Answer from the drawing. Dimensions are ordinates in mm from the lowest x, y and z of the part. Round coordinates to 2 decimals unless told otherwise and drop trailing zeros. Loops run counter-clockwise (first coordinate to the right, second up) from the corner with the lowest first, then second, coordinate; pieces in that order, holes last. Notation, with made-up numbers: (7, 26) - (50, 26) arc R29 cw to (50, 53) - close; hole circle Ø3 at (81, -10.5). An arc over 180 degrees is marked (long way). Answer as CSV lines item,"result".
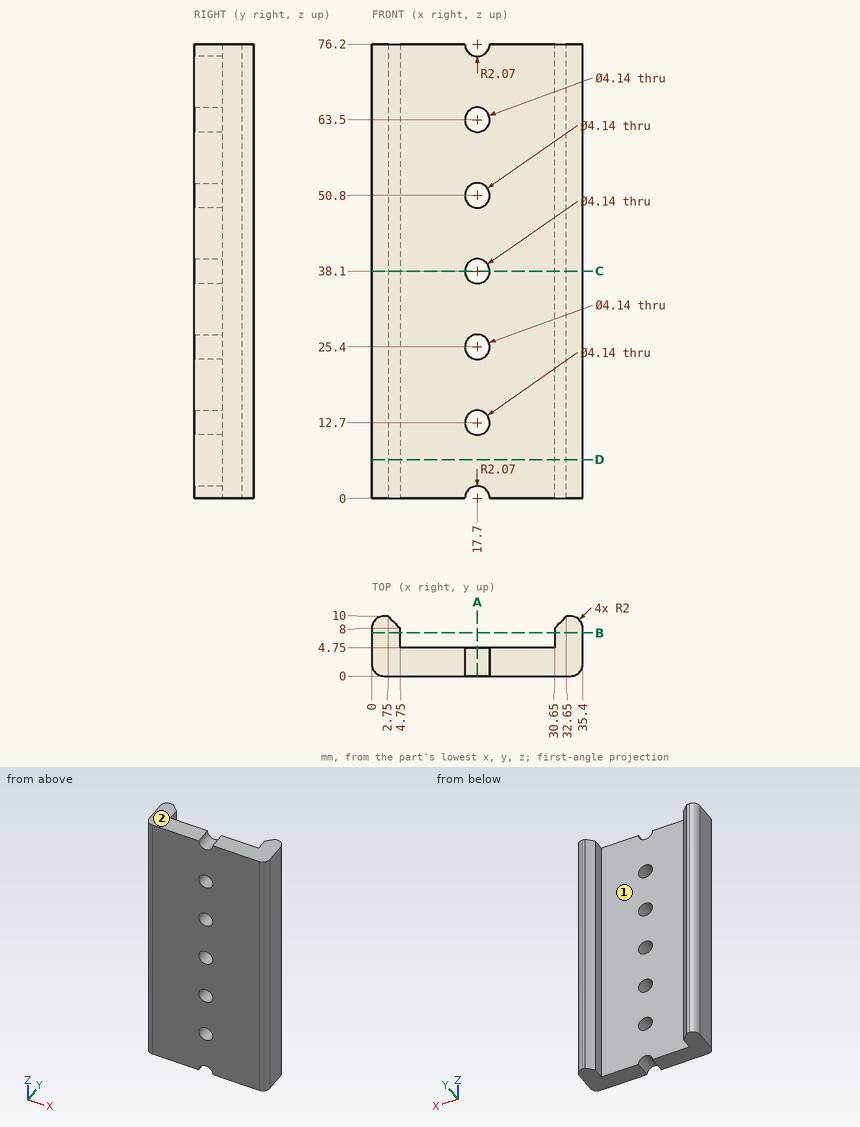
1) A cutting plane is placed at D-D, the plane z = 6.5. Determine the outline of the cut face in (x, y).
Entries:
outline,"(0, 2) arc R2 ccw to (2, 0) - (33.4, 0) arc R2 ccw to (35.4, 2) - (35.4, 8) arc R2 ccw to (33.4, 10) - (32.65, 10) - (30.65, 8) - (30.65, 4.75) - (4.75, 4.75) - (4.75, 8) - (2.75, 10) - (2, 10) arc R2 ccw to (0, 8) - close"
2) The mould has two halves that part along X. Classify the marked faces 1 and 2: pulls with the +X half, pulls with the -X half, needs draft (parallel to the pull), parting line crosses it, or undercut.
Entries:
face 1,"undercut"
face 2,"needs draft"
3) A cutting plane is placed at B-B, the plane y = 7.25. Determine the outline of the cut face in (x, z).
Entries:
outline,"(0, 0) - (4.75, 0) - (4.75, 76.2) - (0, 76.2) - close; (30.65, 0) - (35.4, 0) - (35.4, 76.2) - (30.65, 76.2) - close"
4) A cutting plane is placed at C-C, the plane z = 38.1. Determine the outline of the cut face in (x, y), plus the area to 3 significant figures.
Entries:
outline,"(0, 2) arc R2 ccw to (2, 0) - (15.63, 0) - (15.63, 4.75) - (4.75, 4.75) - (4.75, 8) - (2.75, 10) - (2, 10) arc R2 ccw to (0, 8) - close; (19.77, 0) - (33.4, 0) arc R2 ccw to (35.4, 2) - (35.4, 8) arc R2 ccw to (33.4, 10) - (32.65, 10) - (30.65, 8) - (30.65, 4.75) - (19.77, 4.75) - close"
area,"191 mm^2"
5) Find the intervals of material crossed by line 1 (Z direction, x = 17.7, y = 2.4); line 2 (X direction, y = 7.5, z = 56); line 3 (Z direction, x = 18, y = 3.5), in increasing order.
Entries:
line 1,"z = 2.07 to 10.63, 14.77 to 23.33, 27.47 to 36.03, 40.17 to 48.73, 52.87 to 61.43, 65.57 to 74.13"
line 2,"x = 0 to 4.75, 30.65 to 35.4"
line 3,"z = 2.05 to 10.65, 14.75 to 23.35, 27.45 to 36.05, 40.15 to 48.75, 52.85 to 61.45, 65.55 to 74.15"
6) A cutting plane is placed at A-A, the plane x = 17.7. Determine the outline of the cut face in (y, z).
Entries:
outline,"(0, 2.07) - (4.75, 2.07) - (4.75, 10.63) - (0, 10.63) - close; (0, 14.77) - (4.75, 14.77) - (4.75, 23.33) - (0, 23.33) - close; (0, 27.47) - (4.75, 27.47) - (4.75, 36.03) - (0, 36.03) - close; (0, 40.17) - (4.75, 40.17) - (4.75, 48.73) - (0, 48.73) - close; (0, 52.87) - (4.75, 52.87) - (4.75, 61.43) - (0, 61.43) - close; (0, 65.57) - (4.75, 65.57) - (4.75, 74.13) - (0, 74.13) - close"
7) Each of these flat-tipped pins is pushed along its axis until it touches: P1, Ø2.5, axis at y = 6, z = 47.5, coming from the -X side; P2, Ø13, axis at x = 12, z = 53, coming from the +Y side. Where does it stop, or does it pass through?
Entries:
P1,"stops at x = 0"
P2,"stops at y = 4.75"
